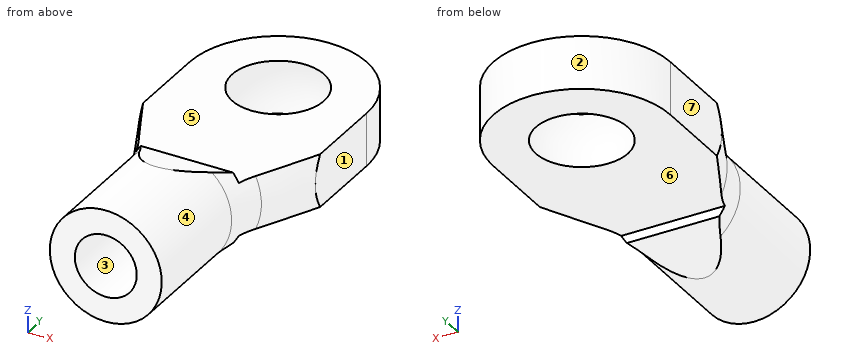
from build123d import *

# Parameters (mm, degrees)
BOSS_EXTRUDE1_DEPTH      = 1.5
BOSS_EXTRUDE1_DEPTH_BACK = 1.5
SKETCH3_R                = 3.5
BOSS_EXTRUDE2_DEPTH      = 8
CUT_EXTRUDE2_DEPTH       = 23.830900114
CUT_EXTRUDE2_DEPTH_BACK  = 23.830900114
SKETCH8_R                = 1.75
CUT_EXTRUDE3_DEPTH       = 5


with BuildPart() as part:
    # Sketch1 → Boss-Extrude1 (new, two sides: drawn at the far end of the back side and taken through both)
    with BuildSketch(Plane.XY.offset(-BOSS_EXTRUDE1_DEPTH_BACK)):
        with BuildLine():
            Line((-3.5, 8.5), (-3.5, 0))
            Line((-3.5, 0), (3.5, 0))
            Line((3.5, 0), (3.5, 8.5))
            Line((3.5, 8.5), (5, 11.8))
            Line((5, 11.8), (5, 17))
            ThreePointArc((5, 17), (0, 22), (-5, 17))
            Line((-5, 17), (-5, 11.8))
            Line((-5, 11.8), (-3.5, 8.5))
        make_face()
    extrude(amount=BOSS_EXTRUDE1_DEPTH + BOSS_EXTRUDE1_DEPTH_BACK)

    # Sketch3 → Boss-Extrude2 (add)
    with BuildSketch(Plane(origin=(0, 0, 0), x_dir=(1, 0, 0), z_dir=(0, 1, 0))):
        Circle(SKETCH3_R)
    extrude(amount=BOSS_EXTRUDE2_DEPTH)

    # Sketch5 → Cut-Extrude2 (cut, two sides: drawn at the far end of the back side and taken through both)
    with BuildSketch(Plane(origin=(0, 0, 0), x_dir=(0, 0, -1), z_dir=(1, 0, 0)).offset(-CUT_EXTRUDE2_DEPTH_BACK)):
        Polygon((2, 8), (3.5, 4), (3.5, 8), align=None)
        Polygon((-3.5, 8), (-2, 8), (-3.5, 4), align=None)
    extrude(amount=CUT_EXTRUDE2_DEPTH + CUT_EXTRUDE2_DEPTH_BACK, mode=Mode.SUBTRACT)

    # Sketch6 → Cut-Revolve1 (revolve, cut)
    with BuildSketch(Plane.XY, mode=Mode.PRIVATE) as cut_revolve1_sk:
        with BuildLine():
            Line((7.363636364, 17), (3.631624104, 9.005417126))
            ThreePointArc((3.631624104, 9.005417126), (3.281024349, 7.973648404), (3.16227766, 6.890428154))
            Line((3.16227766, 6.890428154), (3.16227766, 0))
            Line((3.16227766, 0), (7.363636364, 0))
            Line((7.363636364, 0), (7.363636364, 17))
        make_face()
    revolve(cut_revolve1_sk.sketch.rotate(Axis((0, 0, 0), (0, 1, 0)), 90), axis=Axis((0, 0, 0), (0, 1, 0)), mode=Mode.SUBTRACT)

    # Sketch7 → Cut-Revolve2 (revolve, cut)
    with BuildSketch(Plane.XY):
        with BuildLine():
            Line((0, 20), (0, 14))
            ThreePointArc((0, 14), (3, 17), (0, 20))
        make_face()
    revolve(axis=Axis((0, 0, 0), (0, 1, 0)), mode=Mode.SUBTRACT)

    # Sketch8 → Cut-Extrude3 (cut)
    with BuildSketch(Plane.XZ):
        with Locations(Location((0, 0, 0), (0, 0, 270))):
            Circle(SKETCH8_R)
    extrude(amount=-CUT_EXTRUDE3_DEPTH, mode=Mode.SUBTRACT)


solid = part.part
The listing builds one solid part. Answer for the finished solid, in the listing's coordinates (mm). Face numbers are marked on the shaded views. A direction names the side the tool comes from. Coordinates: 2 decimals unless noted, no trailing zeros. Loops run counter-clockwise (first coordinate to the right, second up) from the corner with the lowest first, then second, coordinate; pieces in that order, holes last.
1) Find section D-D on y = 12.75. Write down the section's boundary in (x, z).
2) A tool of negligible diameter and unlimited length cuts with its end or side. For the marked faces 4, 5, 6 and 7, from which of +Z, -Z, +X, -X, +Y, -Y can it reach the whole face along a straight path? Write none if from no direction.
3) Find section A-A on z = 0. Write down the section's boundary in (x, y), then the cut area to 3 significant figures.
4) Find section C-C on x = 1. Write down the section's boundary in (y, z), then the cut area to 3 significant figures.
5) Find the intervals of material crossed by L1, parallel to X at y = 2.5, z = 0; L2, parallel to Y at x = 1, z = 0.75; L3, parallel to Y at x = 1.25, z = 0.5, in increasing order.
6) Determine the mould class of the marked faces 1, 2 and 3 for opening direction X: pulls with the +X half, pulls with the -X half, needs draft (parallel to the pull), parting line crosses it, or undercut.
7) Find section B-B on y = 15. Write down the section's boundary in (x, z), then the cut area to 3 significant figures.
8) Flat-ended cylindrical pins translate along their axes: pin 1 Ø5 at (x, y) = (4, 8.5) entering from -Z; pin 2 Ø1 at (x, y) = (-1.5, 19) entering from +Z; pin 3 Ø0.6 at (x, z) = (-1, -1.5) entering from +Y; pin 4 Ø4 at (x, y) = (2, 3) entering from +Z. Find the tip coordinate at first contact, or state that the pin passes through.
Values:
1. outline: (-5, -1.5) - (5, -1.5) - (5, 1.5) - (-5, 1.5) - close
2. face 4: -Y
2. face 5: +Z, +X, -X, +Y
2. face 6: -Z, +X, -X, +Y
2. face 7: +Z, -Z, -X, +Y, -Y
3. outline: (-5, 11.94) - (-3.63, 9.01) arc R5 cw to (-3.16, 6.89) - (-3.16, 0) - (-1.75, 0) - (-1.75, 5) - (1.75, 5) - (1.75, 0) - (3.16, 0) - (3.16, 6.89) arc R5 cw to (3.63, 9.01) - (5, 11.94) - (5, 17) arc R5 ccw to (-5, 17) - close; hole circle Ø6 at (0, 17)
3. area: 127 mm2
4. outline: (0, -3) - (5.33, -3) - (8, -2) - (8, -1.5) - (14.6, -1.5) arc R2.83 cw to (14.6, 1.5) - (8, 1.5) - (8, 2) - (5.33, 3) - (0, 3) - (0, 1.44) - (5, 1.44) - (5, -1.44) - (0, -1.44) - close; (19.4, -1.5) - (21.9, -1.5) - (21.9, 1.5) - (19.4, 1.5) arc R2.83 cw to start
4. area: 56.5 mm2
5. L1: x = -3.16 to -1.75, 1.75 to 3.16
5. L2: y = 5 to 14.27, 19.73 to 21.9
5. L3: y = 5 to 14.32, 19.68 to 21.84
6. face 1: pulls with the +X half
6. face 2: parting line crosses it
6. face 3: undercut
7. outline: (-5, -1.5) - (-1.66, -1.5) arc R2.24 cw to (-1.66, 1.5) - (-5, 1.5) - close; (1.66, -1.5) - (5, -1.5) - (5, 1.5) - (1.66, 1.5) arc R2.24 cw to start
7. area: 17.7 mm2
8. pin 1: stops at z = -2.4
8. pin 2: stops at z = 1.5
8. pin 3: stops at y = 21.95
8. pin 4: stops at z = 3.16
